Build history of the part. All positions in model axes, mm. A direction names the side the tool comes from. Give positions to 0.01 mm unless a question says otherwise; leave off trailing zeros. Order: outer loops, then holes, each group sorted by start corner. A loop starts at its lowest first (then second) coordinate and runs counter-clockwise, first axis right, second up. Notation, with made-up numbers: (-24.5, 61) - (17.5, 61) arc R19 ccw to (17.5, 79) - close; hole circle Ø3 at (41, 86). An arc over 180 degrees is marked (long way). One line per item, written item: value.
```python
from build123d import *

# Parameters (mm, degrees)
SKETCH_1_W                = 70
SKETCH_1_H                = 18
EXTRUDE_1_DEPTH           = 60
CUT_EXTRUDE_1_DEPTH       = 94.936148527
SKETCH_3_W                = 15
SKETCH_3_H                = 5
CUT_EXTRUDE_2_DEPTH       = 1
SKETCH_4_W                = 15
SKETCH_4_H                = 5
CUT_EXTRUDE_3_DEPTH       = 1
SKETCH_5_W                = 3
SKETCH_5_H                = 11
CUT_EXTRUDE_4_DEPTH       = 1
SKETCH_6_W                = 3
SKETCH_6_H                = 11
CUT_EXTRUDE_5_DEPTH       = 1
CHAMFER_1_SIZE            = 1
EXTRUDE_9_DEPTH           = 6
SKETCH_7_W                = 29.5
SKETCH_7_H                = 9
CUT_EXTRUDE_7_DEPTH       = 4
SKETCH_9_W                = 37
SKETCH_9_H                = 7.5
EXTRUDE_3_DEPTH           = 12
SKETCH_10_W               = 70
SKETCH_10_H               = 18
EXTRUDE_4_DEPTH           = 8
CHAMFER_4_SIZE            = 4
SKETCH_11_W               = 8
SKETCH_11_H               = 11
CUT_EXTRUDE_8_DEPTH       = 3
SKETCH_12_W               = 0.6
SKETCH_12_H               = 33.5
CUT_EXTRUDE_9_DEPTH       = 13
SKETCH_13_W               = 0.6
SKETCH_13_H               = 52.5
EXTRUDE_5_DEPTH           = 7
SKETCH_14_W               = 0.6
SKETCH_14_H               = 10
EXTRUDE_6_DEPTH           = 1
SKETCH_15_W               = 7.7
SKETCH_15_H               = 49
EXTRUDE_7_DEPTH           = 0.6
SKETCH_18_W               = 7.7
SKETCH_18_H               = 10
EXTRUDE_8_DEPTH           = 0.6
CHAMFER_5_SIZE            = 1.8
SKETCH_22_W               = 3
SKETCH_22_H               = 6.5
CUT_EXTRUDE_10_DEPTH      = 1
EXTRUDE_10_DEPTH          = 18
FILLET_1_R                = 3
HOLE_WIZARD_2_D           = 4.5
HOLE_WIZARD_2_CSINK_D     = 8.6
HOLE_WIZARD_2_CSINK_ANGLE = 90


with BuildPart() as part:
    # 草图1 → 凸台-拉伸1 (new body)
    with BuildSketch(Plane.XY):
        with Locations((35, 9)):
            Rectangle(SKETCH_1_W, SKETCH_1_H)
    extrude(amount=EXTRUDE_1_DEPTH)

    # 草图2 → 切除-拉伸1 (cut, through all)
    with BuildSketch(Plane.XY.offset(60)):
        Polygon((13.4, 0), (13.4, 5), (9.4, 5), (9.4, 12), (60.6, 12), (60.6, 5), (56.6, 5), (56.6, 0), align=None)
    extrude(amount=-CUT_EXTRUDE_1_DEPTH, mode=Mode.SUBTRACT)

    # 草图3 → 切除-拉伸2 (cut)
    with BuildSketch(Plane(origin=(13.4, 0, 0), x_dir=(0, 0, -1), z_dir=(1, 0, 0))):
        with Locations((-7.5, 2.5)):
            Rectangle(SKETCH_3_W, SKETCH_3_H)
    extrude(amount=-CUT_EXTRUDE_2_DEPTH, mode=Mode.SUBTRACT)

    # 草图4 → 切除-拉伸3 (cut)
    with BuildSketch(Plane.ZY.offset(-56.6)):
        with Locations((7.5, 2.5)):
            Rectangle(SKETCH_4_W, SKETCH_4_H)
    extrude(amount=-CUT_EXTRUDE_3_DEPTH, mode=Mode.SUBTRACT)

    # 草图5 → 切除-拉伸4 (cut)
    with BuildSketch(Plane(origin=(0, 5, 0), x_dir=(1, 0, 0), z_dir=(0, 1, 0))):
        with Locations((59.1, -5.5)):
            Rectangle(SKETCH_5_W, SKETCH_5_H)
    extrude(amount=-CUT_EXTRUDE_4_DEPTH, mode=Mode.SUBTRACT)

    # 草图6 → 切除-拉伸5 (cut)
    with BuildSketch(Plane(origin=(0, 5, 0), x_dir=(1, 0, 0), z_dir=(0, 1, 0))):
        with Locations((10.9, -5.5)):
            Rectangle(SKETCH_6_W, SKETCH_6_H)
    extrude(amount=-CUT_EXTRUDE_5_DEPTH, mode=Mode.SUBTRACT)

    # 倒角1
    chamfer_1_edges = [part.edges().sort_by_distance(p)[0] for p in [
        (59.1, 4, 11),
        (10.9, 4, 11),
        (12.4, 2.5, 15),
        (57.6, 2.5, 15),
    ]]
    chamfer(chamfer_1_edges, length=CHAMFER_1_SIZE - 0.0001)  # a hair under: the kernel refuses the full size

    # 草图21 → 凸台-拉伸9 (add)
    with BuildSketch(Plane(origin=(0, 18, 0), x_dir=(1, 0, 0), z_dir=(0, 1, 0))):
        Polygon((0, 0), (16.5, 8), (53.5, 8), (70, 0), align=None)
    extrude(amount=-EXTRUDE_9_DEPTH)

    # 草图7 → 切除-拉伸7 (cut)
    with BuildSketch(Plane.XZ.offset(-12)):
        with Locations((35, 0.5)):
            Rectangle(SKETCH_7_W, SKETCH_7_H)
    extrude(amount=-CUT_EXTRUDE_7_DEPTH, mode=Mode.SUBTRACT)

    # 草图9 → 凸台-拉伸3 (add)
    with BuildSketch(Plane.XZ.offset(-12)):
        with Locations((35, 56.25)):
            Rectangle(SKETCH_9_W, SKETCH_9_H)
    extrude(amount=EXTRUDE_3_DEPTH)

    # 草图10 → 凸台-拉伸4 (add)
    with BuildSketch(Plane.XY.offset(60)):
        with Locations((35, 9)):
            Rectangle(SKETCH_10_W, SKETCH_10_H)
    extrude(amount=EXTRUDE_4_DEPTH)

    # 倒角4
    chamfer_4_edges = [part.edges().sort_by_distance(p)[0] for p in [
        (35, 16, 5),
    ]]
    chamfer(chamfer_4_edges, length=CHAMFER_4_SIZE - 0.0001)  # a hair under: the kernel refuses the full size

    # 草图11 → 切除-拉伸8 (cut)
    with BuildSketch(Plane.XZ):
        with Locations((35, 58)):
            Rectangle(SKETCH_11_W, SKETCH_11_H)
    extrude(amount=-CUT_EXTRUDE_8_DEPTH, mode=Mode.SUBTRACT)

    # 草图12 → 切除-拉伸9 (cut)
    with BuildSketch(Plane.XZ):
        with Locations((22.5, 51.25)):
            Rectangle(SKETCH_12_W, SKETCH_12_H)
        with Locations((47.5, 51.25)):
            Rectangle(SKETCH_12_W, SKETCH_12_H)
    extrude(amount=-CUT_EXTRUDE_9_DEPTH, mode=Mode.SUBTRACT)

    # 草图13 → 凸台-拉伸5 (add)
    with BuildSketch(Plane.XZ.offset(-12)):
        with Locations((16.8, 26.25)):
            Rectangle(SKETCH_13_W, SKETCH_13_H)
        with Locations((53.2, 26.25)):
            Rectangle(SKETCH_13_W, SKETCH_13_H)
    extrude(amount=EXTRUDE_5_DEPTH)

    # 草图14 → 凸台-拉伸6 (add)
    with BuildSketch(Plane.XZ.offset(-5)):
        with Locations((16.8, 5)):
            Rectangle(SKETCH_14_W, SKETCH_14_H)
        with Locations((53.2, 5)):
            Rectangle(SKETCH_14_W, SKETCH_14_H)
    extrude(amount=EXTRUDE_6_DEPTH)

    # 草图15 → 凸台-拉伸7 (add)
    with BuildSketch(Plane.XZ.offset(-5)):
        with Locations((13.25, 35.5)):
            Rectangle(SKETCH_15_W, SKETCH_15_H)
        with Locations((56.75, 35.5)):
            Rectangle(SKETCH_15_W, SKETCH_15_H)
    extrude(amount=EXTRUDE_7_DEPTH)

    # 草图18 → 凸台-拉伸8 (add)
    with BuildSketch(Plane.XZ.offset(-4)):
        with Locations((13.25, 5)):
            Rectangle(SKETCH_18_W, SKETCH_18_H)
        with Locations((56.75, 5)):
            Rectangle(SKETCH_18_W, SKETCH_18_H)
    extrude(amount=EXTRUDE_8_DEPTH)

    # 倒角5
    chamfer_5_edges = [part.edges().sort_by_distance(p)[0] for p in [
        (35, 12, -8),
        (9.4, 12, 30),
        (60.6, 12, 30),
        (6.2, 0, 0),
        (63.8, 0, 0),
    ]]
    chamfer(chamfer_5_edges, length=CHAMFER_5_SIZE)

    # 草图22 → 切除-拉伸10 (cut)
    with BuildSketch(Plane.XZ):
        with Locations((24.3, 60.75)):
            Rectangle(SKETCH_22_W, SKETCH_22_H)
        with Locations((45.7, 60.75)):
            Rectangle(SKETCH_22_W, SKETCH_22_H)
    extrude(amount=-CUT_EXTRUDE_10_DEPTH, mode=Mode.SUBTRACT)

    # 草图23 → 凸台-拉伸10 (add)
    with BuildSketch(Plane(origin=(0, 18, 0), x_dir=(1, 0, 0), z_dir=(0, 1, 0))):
        Polygon((0, -68), (0, -86), (10, -86), (10, -83), (7, -83), (7, -79.7), (10, -79.7), (10, -76.7), (7, -76.7), (7, -68), align=None)
        Polygon((63, -68), (70, -68), (70, -86), (60, -86), (60, -83), (63, -83), (63, -79.7), (60, -79.7), (60, -76.7), (63, -76.7), align=None)
    extrude(amount=-EXTRUDE_10_DEPTH)

    # 圆角1
    fillet_1_edges = [part.edges().sort_by_distance(p)[0] for p in [
        (7, 9, 76.7),
        (7, 9, 68),
        (63, 9, 68),
        (63, 9, 76.7),
    ]]
    fillet(fillet_1_edges, radius=FILLET_1_R - 0.0001)  # a hair under: the kernel refuses the full size

    # 打孔尺寸(%根据十字)槽半沉头木螺钉的类型2 (through all)
    with Locations(Plane(origin=(0, 0, 0), x_dir=(-1, 0, 0), z_dir=(0, -1, 0))):
        with Locations((-65, -12), (-65, -62), (-5, -12), (-5, -62)):
            CounterSinkHole(HOLE_WIZARD_2_D / 2, HOLE_WIZARD_2_CSINK_D / 2, counter_sink_angle=HOLE_WIZARD_2_CSINK_ANGLE)


solid = part.part
```
(1) Slice it at C-C, the plane x = 65. Give the cut face in (y, z), and give its area (3 significant figures).
Completed:
outline: (0, 1.8) - (1.8, 0) - (12, 0) - (12, -2.42) - (18, -2.42) - (18, 9.75) - (2.05, 9.75) - (0, 7.7) - close; (0, 16.3) - (2.05, 14.25) - (18, 14.25) - (18, 59.75) - (2.05, 59.75) - (0, 57.7) - close; (0, 66.3) - (2.05, 64.25) - (18, 64.25) - (18, 86) - (0, 86) - close
area: 1,390 mm²
(2) Pull direction Z, two halves, no side cores. Call faces 4 (the face through (35, 9, 68)), 5 (the face through (61.63, 15.04, -4.06)), 6 (the face through (55, 3.4, 5)), 7 (the face through (20.25, 14, -1)): +Z half, -Z half, draft (parallel to the pull), parting line (faces both ways), or undercut.
Completed:
face 4: +Z half
face 5: -Z half
face 6: draft
face 7: undercut
(3) 3-axis set-ups, long thin cutter, end or side, ignore diameter. For faces 1 (the face through (65, 7, 0)), 2 (the face through (8, 9, 79.7)), 3 (the face through (16.5, 8, 30)): which of +Z, -Z, +X, -X, +Y, -Y reach the whole face in a straight line?
Completed:
face 1: -Z, +X, -X, -Y
face 2: +Y, -Y
face 3: -Z
(4) Slice it at A-A, the plane z = 12. Count the separate pieces of the cut face and the enclosed holes in it, and give its area (3 significant figures).
Completed:
separate pieces: 3
enclosed holes: 2
area: 522 mm²
(5) Drill centre lines: line 1 (Z direction, x = 6, y = 3.75); line 2 (X direction, y = 6.25, z = 62); line 3 (X direction, y = 8.5, z = 47.5). Where is each one in solid material? Low to high.
Completed:
line 1: 0 to 9.98, 14.02 to 59.98, 64.02 to 86
line 2: 0 to 2.75, 7.25 to 22.2, 22.8 to 47.2, 47.8 to 62.75, 67.25 to 70
line 3: 0 to 9.4, 16.5 to 17.1, 52.9 to 53.5, 60.6 to 70
(6) Pin check, flat tips, straight feed: P1, Ø10, axis at x = 34, y = 6.5, coming from the -Z side; P2, Ø1.5, axis at x = 42.5, y = 7.5, coming from the +Z side; P3, Ø2.5, axis at x = 5, z = 12, coming from the +Y side; P4, Ø1.6, axis at x = 54.5, y = 2, coming from the -Z side. Stop position of each tip, or through.
Completed:
P1: z = 52.5
P2: z = 68
P3: through
P4: z = 60
